from build123d import *

# Parameters (mm, degrees)
SKETCH_1_R          = 16.5
EXTRUDE_1_DEPTH     = 23
SKETCH_2_R          = 4.125
EXTRUDE_2_DEPTH     = 1
SKETCH_3_R          = 1
EXTRUDE_3_DEPTH     = 8
SKETCH_4_R          = 3
EXTRUDE_4_DEPTH     = 2
EXTRUDE_START       = 8.5
SKETCH_5_R          = 16.5
EXTRUDE_5_DEPTH     = 8.5
SKETCH_6_R          = 1.3
CUT_EXTRUDE_1_DEPTH = 2


with BuildPart() as part:
    # 草图1 → 凸台-拉伸1 (new body)
    with BuildSketch(Plane(origin=(0, 0, 0), x_dir=(1, 0, 0), z_dir=(0, 1, 0))):
        with Locations(Location((0, 0, 0), (0, 0, 270))):
            Circle(SKETCH_1_R)
    extrude(amount=EXTRUDE_1_DEPTH)

    # 草图2 → 凸台-拉伸2 (add)
    with BuildSketch(Plane(origin=(0, 23, 0), x_dir=(1, 0, 0), z_dir=(0, 1, 0))):
        with Locations(Location((0, 0, 0), (0, 0, 270))):
            Circle(SKETCH_2_R)
    extrude(amount=EXTRUDE_2_DEPTH)

    # 草图3 → 凸台-拉伸3 (add)
    with BuildSketch(Plane(origin=(0, 24, 0), x_dir=(1, 0, 0), z_dir=(0, 1, 0))):
        with Locations(Location((0, 0, 0), (0, 0, 270))):
            Circle(SKETCH_3_R)
    extrude(amount=EXTRUDE_3_DEPTH)

    # 草图4 → 凸台-拉伸4 (add)
    with BuildSketch(Plane.XZ):
        with Locations(Location((0, 0, 0), (0, 0, 90))):
            Circle(SKETCH_4_R)
    extrude(amount=EXTRUDE_4_DEPTH)

    # 草图5 → 凸台-拉伸5 (add)
    with BuildSketch(Plane(origin=(0, -2, 0), x_dir=(-1, 0, 0), z_dir=(0, -1, 0)).offset(EXTRUDE_START)):
        with Locations(Location((0, 0, 0), (0, 0, 270))):
            Circle(SKETCH_5_R)
    extrude(amount=-EXTRUDE_5_DEPTH)

    # 草图6 → 切除-拉伸1 (cut)
    with BuildSketch(Plane(origin=(0, 23, 0), x_dir=(1, 0, 0), z_dir=(0, 1, 0))):
        with Locations(Location((-11.258330249, -6.5, 0), (0, 0, 270))):
            Circle(SKETCH_6_R)
        with Locations(Location((0, -13, 0), (0, 0, 270))):
            Circle(SKETCH_6_R)
        with Locations(Location((11.258330249, -6.5, 0), (0, 0, 270))):
            Circle(SKETCH_6_R)
        with Locations(Location((11.258330249, 6.5, 0), (0, 0, 270))):
            Circle(SKETCH_6_R)
        with Locations(Location((0, 13, 0), (0, 0, 270))):
            Circle(SKETCH_6_R)
        with Locations(Location((-11.258330249, 6.5, 0), (0, 0, 270))):
            Circle(SKETCH_6_R)
    extrude(amount=-CUT_EXTRUDE_1_DEPTH, mode=Mode.SUBTRACT)


solid = part.part
Design review of the part built by this model. Coordinates are the model's own, in mm. A direction names the side the tool comes from. Round coordinates to 2 decimals unless told otherwise and drop trailing zeros. Order: outer loops, then holes, each group sorted by start corner. A loop starts at its lowest first (then second) coordinate and runs counter-clockwise, first axis right, second up. Notation, with made-up numbers: M -10.75,55 L 47.25,55 A10 ccw 47.25,65 Z; hole C 33,32.25 d8. An arc over 180 degrees is marked long. Answer as CSV lines item,"result". Start each with the question number.
1) Wall thickness on line 1 along Y through (x, z) = (-13.5, -3.5); line 2 along Y through (x, z) = (11, 7); line 3 along X through (y, z) = (22, -6): over which ranges is each line inside the solid? List them lowest first. Write a range as [from, to].
2) Add section C-C (z = 0). Give the boundary of the cut face in (x, y) (3 decimals), then the cut area to 3 significant figures.
3) Tool access review of faces 1 (the face through (-12.41, 22.01, 7.1)), 2 (the face through (0, -10.5, 0)), 3 (the face through (-0.9, -0.99, 2.86)): name each direction out of +Z, -Z, +X, -X, +Y, -Y from which nothing blocks a thin tool from reaching the whole face with its end or side.
4) Add section B-B (x = -5.5). Give the boundary of the cut face in (y, z), then the cut area to 3 significant figures.
5) The part is to be moulded in two halves that separate along X. For faces 4 (the face through (-3.4, 0, -0.2)), 5 (the face through (16.108, -6.31, -3.577)), 6 (the face through (-11, 21, -7)), say which applies: +X half, -X half, draft (parallel to the pull), parting line (faces both ways), or undercut.
6) Add section D-D (x = 0). Give the boundary of the cut face in (y, z) (3 decimals), then the cut area to 3 significant figures.
7) Add section A-A (z = -6). Give the boundary of the cut face in (x, y), then the cut area to 3 significant figures.
8) For pin 1 Ø2 at (x, z) = (-11, -7) entering from +Y; pin 2 Ø4 at (x, y) = (-5, 26) entering from -Z; pin 3 Ø10 at (y, z) = (23, -1) entering from -X; pin 4 Ø12 at (y, z) = (7, -9.5) entering from -X, all flat-tipped, find the tip position at first contact; note any pin that passes through.
Resolved:
1,line 1,"[-10.5, -2], [0, 23]"
1,line 2,"[-10.5, -2], [0, 21]"
1,line 3,"[-15.37, -12.46], [-10.06, 10.06], [12.46, 15.37]"
2,outline,"M -16.5,-10.5 L 16.5,-10.5 L 16.5,-2 L 3,-2 L 3,0 L 16.5,0 L 16.5,23 L 4.125,23 L 4.125,24 L 1,24 L 1,32 L -1,32 L -1,24 L -4.125,24 L -4.125,23 L -16.5,23 L -16.5,0 L -3,0 L -3,-2 L -16.5,-2 Z"
2,area,"1,080 mm^2"
3,face 1,"+Y"
3,face 2,"+Z, -Z, +X, -X, -Y"
3,face 3,"none"
4,outline,"M -10.5,-15.56 L -2,-15.56 L -2,15.56 L -10.5,15.56 Z; M 0,-15.56 L 23,-15.56 L 23,15.56 L 0,15.56 Z"
4,area,"980 mm^2"
5,face 4,"draft"
5,face 5,"parting line"
5,face 6,"undercut"
6,outline,"M -10.5,-16.5 L -2,-16.5 L -2,-3 L 0,-3 L 0,-16.5 L 23,-16.5 L 23,-14.3 L 21,-14.3 L 21,-11.7 L 23,-11.7 L 23,-4.125 L 24,-4.125 L 24,-1 L 32,-1 L 32,1 L 24,1 L 24,4.125 L 23,4.125 L 23,11.7 L 21,11.7 L 21,14.3 L 23,14.3 L 23,16.5 L 0,16.5 L 0,3 L -2,3 L -2,16.5 L -10.5,16.5 Z"
6,area,"1,070 mm^2"
7,outline,"M -15.37,-10.5 L 15.37,-10.5 L 15.37,-2 L -15.37,-2 Z; M -15.37,0 L 15.37,0 L 15.37,23 L 12.46,23 L 12.46,21 L 10.06,21 L 10.06,23 L -10.06,23 L -10.06,21 L -12.46,21 L -12.46,23 L -15.37,23 Z"
7,area,"959 mm^2"
8,pin 1,"y = 23"
8,pin 2,"through"
8,pin 3,"x = -16.5"
8,pin 4,"x = -16.12"
